Check sheet for the modelled part. Datum: model origin and axes. Units: mm. A direction names the side the tool comes from. Round coordinates to 2 decimals unless told otherwise and drop trailing zeros. Write each loop counter-clockwise with the first axis right and the second up, starting at its lowest first coordinate (ties: lowest second). Pieces come first, ordered by that corner, then holes.
Item 1: Go/stop test with flat-tipped pins: pin 1 Ø2 at (x, z) = (-32, -9) entering from +Y; pin 2 Ø1.1 at (y, z) = (-1, -7.5) entering from +X; pin 3 Ø1.5 at (x, z) = (84.5, -8) entering from +Y. Record where each tip stops, or that it passes through.
Item 2: Release check for a two-part mould opening along X. For faces 1 (the flat face through (123.505, -2, -10)), 2 (the flat face through (13.505, -2, -10)), 3 (the flat face through (-0.495, 7.4, 4.5)) record: +X half, -X half, draft (parallel to the pull), parting line (faces both ways), or undercut.
Item 3: Material ranges on line 1 (X direction, y = -2.25, z = 9.5); line 2 (X direction, y = 8.25, z = -3.5); line 3 (Y direction, x = 170, z = 0.5), recorded low to high.
Item 4: Cross-section at B-B on x = -31.5. Enter the section's corners in (y, z).
Item 5: Tool access check on faces 4 (the cylindrical face through (162.71, -3, -9.54)), 5 (the cylindrical face through (0.519, -8.428, 1.107)), 6 (the flat face through (-55, 0, 6.278)). Record the directions out of +Z, -Z, +X, -X, +Y, -Y that give a thin tool (end or side, any length) a straight path to the whole face; none if there is none.
Item 6: Cross-section at A-A on z = 0. Enter the section's corners in (x, y), plus the area to 3 significant figures.
Item 7: Cross-section at C-C on x = 64. Enter the section's corners in (y, z) (1 decimal).
from build123d import *

# Parameters (mm, degrees)
CORTAR_EXTRUIR1_START = -23
CORTAR_EXTRUIR1_DEPTH = 23


with BuildPart() as part:
    # Croquis1 → Revolución1 (revolve)
    with BuildSketch(Plane.XY, mode=Mode.PRIVATE) as revoluci_n1_sk:
        Polygon((13.505191192, 11.1125), (68.505191192, 11.1125), (68.505191192, 0), (-66.494808808, 0), (-66.494808808, 10), (-0.494808808, 10), (-0.494808808, 8.5), (1.505191192, 8.5), (1.505191192, 10), (13.505191192, 10), align=None)
    revoluci_n1 = revolve(revoluci_n1_sk.sketch.rotate(Axis((70.414965315, 0, 0), (-1, 0, 0)), 90), axis=Axis((70.414965315, 0, 0), (-1, 0, 0)))

    # Croquis2 → Cortar-Extruir1 (cut)
    with BuildSketch(Plane.ZY.offset(66.494808808).offset(CORTAR_EXTRUIR1_START)):
        with BuildLine():
            Line((-6.278365003, -7.783452504), (-6.278365003, 7.783452504))
            ThreePointArc((-6.278365003, 7.783452504), (-10, 0), (-6.278365003, -7.783452504))
        make_face()
        with BuildLine():
            Line((6.278365003, -7.783452504), (6.278365003, 7.783452504))
            ThreePointArc((6.278365003, 7.783452504), (10, 0), (6.278365003, -7.783452504))
        make_face()
    cortar_extruir1 = extrude(amount=CORTAR_EXTRUIR1_DEPTH, mode=Mode.SUBTRACT)

    # Simetría2: Revolución1, Cortar-Extruir1 across plane
    add(revoluci_n1.mirror(Plane(origin=(68.505191192, 11.1125, 0), x_dir=(0, 0, 1), z_dir=(1, 0, 0))))
    add(cortar_extruir1.mirror(Plane(origin=(68.505191192, 11.1125, 0), x_dir=(0, 0, 1), z_dir=(1, 0, 0))), mode=Mode.SUBTRACT)


solid = part.part
Response values:
1. pin 1: stops at y = 6
1. pin 2: stops at x = 180.51
1. pin 3: stops at y = 8.42
2. face 1: +X half
2. face 2: -X half
2. face 3: undercut
3. line 1: x = -43.49 to -0.49, 1.51 to 135.51, 137.51 to 180.51
3. line 2: x = -66.49 to -0.49, 1.51 to 135.51, 137.51 to 203.51
3. line 3: y = -9.99 to 9.99
4. outline: circle Ø20 at (0, 0)
5. face 4: +X
5. face 5: none
5. face 6: +Z, -X, +Y, -Y
6. outline: (-66.49, -10) - (-0.49, -10) - (-0.49, -8.5) - (1.51, -8.5) - (1.51, -10) - (13.51, -10) - (13.51, -11.11) - (123.51, -11.11) - (123.51, -10) - (135.51, -10) - (135.51, -8.5) - (137.51, -8.5) - (137.51, -10) - (203.51, -10) - (203.51, 10) - (137.51, 10) - (137.51, 8.5) - (135.51, 8.5) - (135.51, 10) - (123.51, 10) - (123.51, 11.11) - (13.51, 11.11) - (13.51, 10) - (1.51, 10) - (1.51, 8.5) - (-0.49, 8.5) - (-0.49, 10) - (-66.49, 10) - close
6. area: 5,630 mm2
7. outline: circle Ø22.2 at (0, 0)
